from build123d import *

# Parameters (mm, degrees)
EXTRUDE_1_DEPTH     = 26
FILLET_1_R          = 1.25
SKETCH_17_R         = 22.5
SKETCH_17_R_2       = 21.415
EXTRUDE_2_DEPTH     = 1.5
CHAMFER_1_SIZE      = 1.5
SKETCH_18_R         = 28.867513459
CUT_EXTRUDE_2_DEPTH = 47.198845585
FILLET_2_R          = 0.5
CHAMFER_2_SIZE      = 1
SKETCH_19_OUTSIDE_W = 75.872
SKETCH_19_OUTSIDE_H = 68.136
SKETCH_19_OUTSIDE_R = 28
CUT_EXTRUDE_4_DEPTH = 47.198845585
CHAMFER_3_SIZE      = 2.5


# Some blends are built 0.0001 mm under size
with BuildPart() as part:
    # Эскиз1 → Бобышка-Вытянуть1 (new body)
    with BuildSketch(Plane.XY):
        Polygon((28.867513459, 0), (14.43375673, 25), (-14.43375673, 25), (-28.867513459, 0), (-14.43375673, -25), (14.43375673, -25), align=None)
    extrude(amount=-EXTRUDE_1_DEPTH)

    # Sketch 4 → Вырез-Повернуть1 (revolve, cut)
    with BuildSketch(Plane(origin=(0, 0, 0), x_dir=(1, 0, 0), z_dir=(0, 1, 0)), mode=Mode.PRIVATE) as cut_revolve_1_sk:
        Polygon((-28.867513459, 26), (-28.867513459, 23.5), (-24.537386441, 26), align=None)
        Polygon((-28.867513459, 0), (-28.867513459, 2.5), (-24.537386441, 0), align=None)
    revolve(cut_revolve_1_sk.sketch.rotate(Axis((0, 0, 0), (0, 0, -1)), 180.000000003), axis=Axis((0, 0, 0), (0, 0, -1)), mode=Mode.SUBTRACT)

    # Эскиз5 → Вырез-Повернуть2 (revolve, cut)
    with BuildSketch(Plane(origin=(0, 0, 0), x_dir=(1, 0, 0), z_dir=(0, 1, 0))):
        Polygon((0, 0), (-22.5, 0), (-22.5, 14.8), (-22.9, 15.2), (-22.9, 17.8), (-21.5, 17.8), (-21.5, 21.1), (-20.25, 21.1), (-20.25, 26), (0, 26), align=None)
    revolve(axis=Axis((0, 0, -26), (0, 0, 1)), mode=Mode.SUBTRACT)

    # Скругление1
    fillet_1_edges = [part.edges().sort_by_distance(p)[0] for p in [
        (21.5, 0, -21.1),
    ]]
    fillet(fillet_1_edges, radius=FILLET_1_R - 0.0001)  # a hair under: the kernel refuses the full size

    # Скругление2
    fillet_2_edges = [part.edges().sort_by_distance(p)[0] for p in [
        (22.9, 0, -17.8),
        (21.5, 0, -17.8),
    ]]
    fillet(fillet_2_edges, radius=FILLET_2_R)

    # Фаска2
    chamfer_2_edges = [part.edges().sort_by_distance(p)[0] for p in [
        (20.25, 0, -26),
    ]]
    chamfer(chamfer_2_edges, length=CHAMFER_2_SIZE)

    # Эскиз19 outside → Вырез-Вытянуть4 (cut, through all)
    with BuildSketch(Plane(origin=(0, 0, -26), x_dir=(-1, 0, 0), z_dir=(0, 0, -1))):
        Rectangle(SKETCH_19_OUTSIDE_W, SKETCH_19_OUTSIDE_H)
        Circle(SKETCH_19_OUTSIDE_R, mode=Mode.SUBTRACT)
    extrude(amount=-CUT_EXTRUDE_4_DEPTH, mode=Mode.SUBTRACT)

    # Фаска3
    # the kernel refuses this chamfer: 2.5 mm, written as the material it takes off along each edge
    with BuildSketch(Plane(origin=(0, 0, 0), x_dir=(-1, 0, 0), z_dir=(0, 1, 0))) as chamfer_3_piece_1:
        Polygon((22.5, -CHAMFER_3_SIZE), (22.5 + CHAMFER_3_SIZE, 0), (22.5, 0), align=None)
    revolve(axis=Axis((0, 0, 0), (0, 0, 1)), mode=Mode.SUBTRACT)


with BuildPart() as body_2:
    # Эскиз17 → Бобышка-Вытянуть2 (new body)
    with BuildSketch(Plane.XY):
        with Locations(Location((0, 0, 0), (0, 0, 180))):
            Circle(SKETCH_17_R)
        Circle(SKETCH_17_R_2, mode=Mode.SUBTRACT)
    extrude(amount=EXTRUDE_2_DEPTH)

    # Фаска1
    # the kernel refuses this chamfer: 1.5 mm, written as the material it takes off along each edge
    with BuildSketch(Plane(origin=(0, 0, 1.5), x_dir=(1, 0, 0), z_dir=(0, -1, 0))) as chamfer_1_piece_1:
        Polygon((21.415, -CHAMFER_1_SIZE), (21.415 + CHAMFER_1_SIZE, 0), (21.415, 0), align=None)
    revolve(axis=Axis((0, 0, 1.5), (0, 0, 1)), mode=Mode.SUBTRACT)

    # Эскиз18 → Вырез-Вытянуть2 (cut, through all)
    with BuildSketch(Plane.XY):
        Circle(SKETCH_18_R)
    extrude(amount=CUT_EXTRUDE_2_DEPTH, mode=Mode.SUBTRACT)


solid = part.part
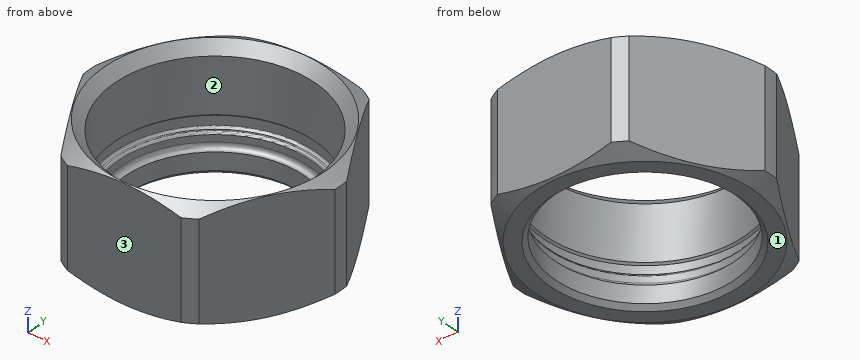
Work out the finished part from the listing and answer in its coordinate system (mm). Face numbers are marked on the shaded views. Round coordinates to 2 decimals unless told otherwise and drop trailing zeros. Order: outer loops, then holes, each group sorted by start corner. A loop starts at its lowest first (then second) coordinate and runs counter-clockwise, first axis right, second up. Notation, with made-up numbers: M 40.25,83.5 L 84.25,83.5 A8 ccw 84.25,89.5 Z; hole C 42.25,77.5 d7. An arc over 180 degrees is marked long. Put each result on its own line as item: value. Start each with the question number.
Q1. Section C-C, the plane z = -6.25 is taken. Write down the section's boundary in (x, y).
Q2. Straight lines are drawn through the part: L1, parallel to Y at x = 0, z = -8; L2, parallel to Y at x = 0, z = -18.65; L3, parallel to X at y = -14, z = -6.25. For each, find the intervals that lie inside material, in ascending order. Write a range as [from, to].
Q3. Flat-ended cylindrical pins translate along their axes: pin 1 (1.5 mm diameter, centred on y = 7, z = -20, fed in from -X); pin 2 (2 mm diameter, centred on x = -18, z = -15, fed in from +Y). Find the tip coordinate at first contact, or state that the pin passes through.
Q4. For a pull along Y with two mould halves and no side action, classify the marked faces 1, 2 and 3 as pulls with the +Y half, pulls with the -Y half, needs draft (parallel to the pull), parting line crosses it, or undercut.
Findings below:
1. outline: M -27.96,-1.58 L -15.35,-23.42 A28 ccw -12.61,-25 L 12.61,-25 A28 ccw 15.35,-23.42 L 27.96,-1.58 A28 ccw 27.96,1.58 L 15.35,23.42 A28 ccw 12.61,25 L -12.61,25 A28 ccw -15.35,23.42 L -27.96,1.58 A28 ccw Z; hole C 0,0 d45
2. L1: y = [-25, -22.5], [22.5, 25]
2. L2: y = [-25, -21.5], [21.5, 25]
2. L3: x = [-20.78, -17.61], [17.61, 20.78]
3. pin 1: stops at x = -25.26
3. pin 2: stops at y = 20.56
4. face 1: needs draft
4. face 2: undercut
4. face 3: pulls with the -Y half
